The listing builds one solid part. Answer for the finished solid, in the listing's coordinates (mm). A direction names the side the tool comes from. Give positions to 0.01 mm unless a question says otherwise; leave off trailing zeros. Write each loop counter-clockwise with the first axis right and the second up, starting at its lowest first coordinate (ties: lowest second). Pieces come first, ordered by that corner, then holes. Notation, with made-up numbers: (-30, 32) -> (11, 32) arc R25 ccw to (11, 59) -> close; hole circle Ø5 at (-32, 7.25). An arc over 180 degrees is marked (long way). Put each result on its own line as item: value. Start each with the question number.
1) A cutting plane is placed at B-B (z = -13). Write down the section's boundary in (x, y).
2) A cutting plane is placed at D-D (x = -14). Write down the section's boundary in (y, z), then the cut area to 3 significant figures.
3) A cutting plane is placed at A-A (x = 0). Write down the section's boundary in (y, z) (3 decimals), then the cut area to 3 significant figures.
4) For faces 4 (the flat face through (0, -2.54, 0)), 5 (the cylindrical face through (-10.074, -5.044, -1.323)), 6 (the cylindrical face through (-14.56, -1.25, -0.41)), determine the directions among +Z, -Z, +X, -X, +Y, -Y from which every point of the face is accessible in a straight line to the end or side of a thin tool.
5) For a pull along X with two mould halves and no side action, classify faces 1 (the cylindrical face through (-11.59, -1.25, -15.12)), 2 (the flat face through (-6, -10.16, -3)), 3 (the cylindrical face through (-3.86, -1.25, -5.04)) as released by +X, released by -X, zero draft, split by the parting line, or undercut.
6) Find the intervals of material crossed by line 1 along X through (y, z) = (-0.95, 0) (3 decimals); line 2 along Y through (x, z) = (1, -15.5); line 3 along Z through (x, y) = (13.5, -1), in increasing order. Write a range as from..to.
7) Flat-ended cylindrical pins translate along their axes: pin 1 Ø1 at (y, z) = (-2.5, 4.5) entering from -X; pin 2 Ø3 at (x, y) = (9, -5) entering from +Z; pin 3 Ø2 at (x, y) = (-3, -5.5) entering from +Z. Find the tip coordinate at first contact, or state that the pin passes through.
8) A cutting plane is placed at C-C (y = -1.5). Write down the section's boundary in (x, z) (3 decimals), then the cut area to 3 significant figures.
from build123d import *

# Parameters (mm, degrees)
SKETCH2_R           = 19.05
SKETCH2_R_2         = 6.35
SKETCH2_R_3         = 1.905
BOSS_EXTRUDE1_DEPTH = 2.54
SKETCH3_R           = 10.16
BOSS_EXTRUDE2_DEPTH = 7.62
FILLET1_R           = 2.54


with BuildPart() as part:
    # Sketch2 → Boss-Extrude1 (new body)
    with BuildSketch(Plane(origin=(0, 0, 0), x_dir=(1, 0, 0), z_dir=(0, 1, 0))):
        with Locations(Location((0, 0, 0), (0, 0, 270))):
            Circle(SKETCH2_R)
        with Locations(Location((0, 0, 0), (0, 0, 270))):
            Circle(SKETCH2_R_2, mode=Mode.SUBTRACT)
        with Locations(Location((0, 12.7, 0), (0, 0, 270))):
            Circle(SKETCH2_R_3, mode=Mode.SUBTRACT)
        with Locations(Location((12.7, 0, 0), (0, 0, 270))):
            Circle(SKETCH2_R_3, mode=Mode.SUBTRACT)
        with Locations(Location((0, -12.7, 0), (0, 0, 270))):
            Circle(SKETCH2_R_3, mode=Mode.SUBTRACT)
        with Locations(Location((-12.7, 0, 0), (0, 0, 270))):
            Circle(SKETCH2_R_3, mode=Mode.SUBTRACT)
    extrude(amount=-BOSS_EXTRUDE1_DEPTH)

    # Sketch3 → Boss-Extrude2 (add)
    with BuildSketch(Plane.XZ.offset(2.54)):
        with Locations(Location((0, 0, 0), (0, 0, 90))):
            Circle(SKETCH3_R)
    extrude(amount=BOSS_EXTRUDE2_DEPTH)

    # Fillet1
    fillet1_edges = [part.edges().sort_by_distance(p)[0] for p in [
        (0, -10.16, -10.16),
    ]]
    fillet(fillet1_edges, radius=FILLET1_R)


with BuildPart() as body_2:
    # Sketch5 → Revolve1 (revolve)
    with BuildSketch(Plane.XZ.offset(10.16)):
        with BuildLine():
            Line((0, 6.35), (0, -6.35))
            ThreePointArc((0, -6.35), (6.35, 0), (0, 6.35))
        make_face()
    revolve(axis=Axis((0, -10.16, -11.766022755), (0, 0, 1)))


with BuildPart() as part_1:
    add(part.part)

    # Combine1: cut body 2
    add(body_2.part, mode=Mode.SUBTRACT)


solid = part_1.part
Reply:
1. outline: (-13.92, -2.54) -> (-1.88, -2.54) -> (-1.88, 0) -> (-13.92, 0) -> close; (1.88, -2.54) -> (13.92, -2.54) -> (13.92, 0) -> (1.88, 0) -> close
2. outline: (-2.54, -12.92) -> (0, -12.92) -> (0, -1.39) -> (-2.54, -1.39) -> close; (-2.54, 1.39) -> (0, 1.39) -> (0, 12.92) -> (-2.54, 12.92) -> close
2. area: 58.6 mm2
3. outline: (-10.16, -7.62) arc R2.54 ccw to (-7.62, -10.16) -> (-2.54, -10.16) -> (-2.54, -10.795) -> (0, -10.795) -> (0, -6.35) -> (-2.54, -6.35) -> (-2.54, 6.35) -> (0, 6.35) -> (0, 10.795) -> (-2.54, 10.795) -> (-2.54, 10.16) -> (-7.62, 10.16) arc R2.54 ccw to (-10.16, 7.62) -> (-10.16, 6.35) arc R6.35 cw to (-10.16, -6.35) -> close; (-2.54, -19.05) -> (0, -19.05) -> (0, -14.605) -> (-2.54, -14.605) -> close; (-2.54, 14.605) -> (0, 14.605) -> (0, 19.05) -> (-2.54, 19.05) -> close
3. area: 134 mm2
4. face 4: +Y
4. face 5: -Y
4. face 6: +Y, -Y
5. face 1: split by the parting line
5. face 2: zero draft
5. face 3: undercut
6. line 1: x = -19.05..-14.605, -10.795..-6.35, 6.35..10.795, 14.605..19.05
6. line 2: y = -2.54..0
6. line 3: z = -13.44..-1.73, 1.73..13.44
7. pin 1: stops at x = -18.63
7. pin 2: stops at z = 6.85
7. pin 3: stops at z = 9.96
8. outline: circle Ø38.1 at (0, 0); hole circle Ø3.81 at (-12.7, 0); hole circle Ø12.7 at (0, 0); hole circle Ø3.81 at (0, -12.7); hole circle Ø3.81 at (0, 12.7); hole circle Ø3.81 at (12.7, 0)
8. area: 968 mm2
